Geometry check sheet. Reference: drawing and pictorial views, mm from the part's lowest x, y, z. A direction names the side the tool comes from. Round coordinates to 2 decimals unless told otherwise and drop trailing zeros. Order: outer loops, then holes, each group sorted by start corner. A loop starts at its lowest first (then second) coordinate and runs counter-clockwise, first axis right, second up.
(1) Tool access check on the marked faces 1 and 2. Record the directions out of +Z, -Z, +X, -X, +Y, -Y that give a thin tool (end or side, any length) a straight path to the whole face; none if there is none.
(2) Mould release check, pull along X, two halves, no side actions. Record for the marked faces 3, 4 and 5: released by +X, released by -X, zero draft, split by the parting line, or undercut.
(3) Thickness scan on probe 1 along X at (y, z) = (27, 8.5); probe 2 along Z at (x, y) = (1.15, 46.5); probe 3 along Y at (x, z) = (13, 3.25). Record the ranges inside material, lowest first.
(4) Sectioned sample at C-C, the plane z = 17. Enter the section's corners in (x, y).
(5) Depth check by flat-ended pin: pin 1 (12 mm diameter, centred on x = 29, z = 3.5, fed in from -Y); pin 2 (3.5 mm diameter, centred on y = 57, z = 10.25, fed in from -X); pin 3 (6 mm diameter, centred on x = 13, z = 15, fed in from +Y). Enter the tip coordinate at first touch or a pass-through.
(6) Sectioned sample at D-D, the plane y = 15.5. Enter the section's corners in (x, z).
(7) Sectioned sample at B-B, the plane y = 23.5. Enter the section's corners in (x, z), and give its area (3 significant figures).
(8) Sectioned sample at A-A, the plane y = 57. Enter the section's corners in (x, z) (3 decimals).
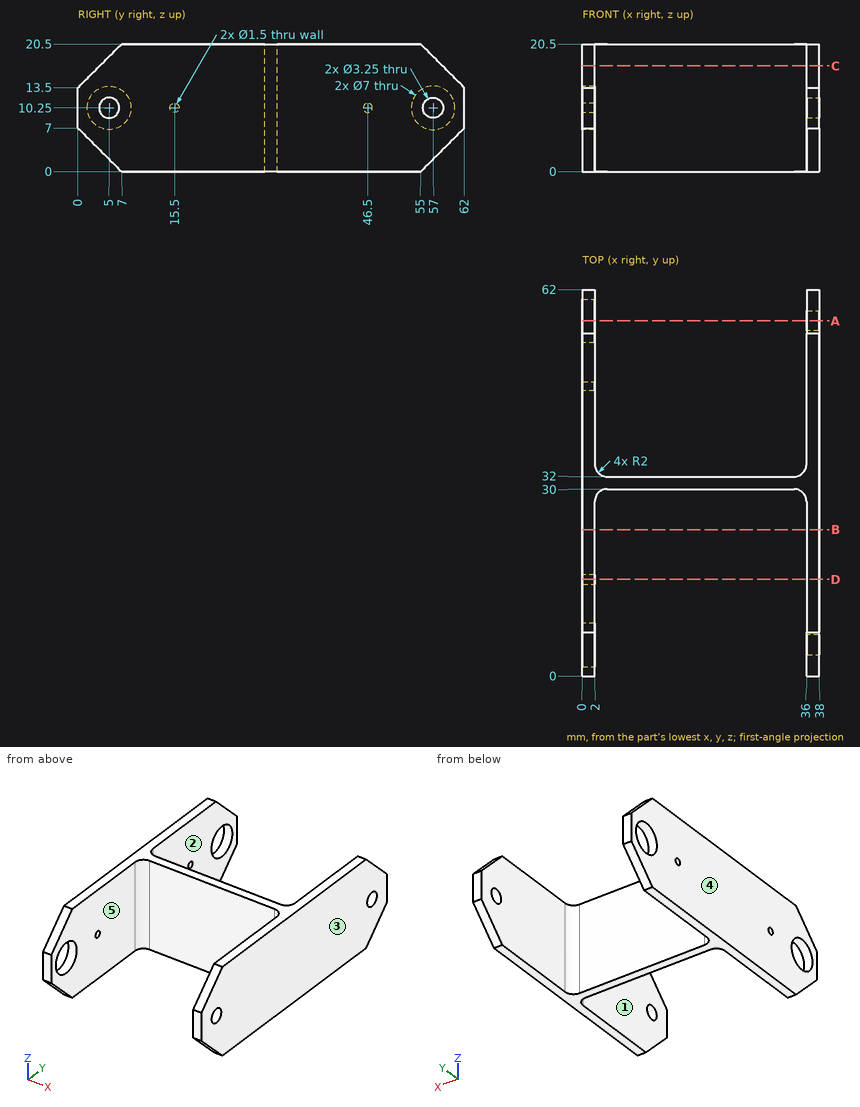
Derived:
1. face 1: +Z, -Z, -Y
1. face 2: +Z, -Z, +Y
2. face 3: released by +X
2. face 4: released by -X
2. face 5: undercut
3. probe 1: x = 0 to 2, 36 to 38
3. probe 2: z = 0 to 9.5, 11 to 20.5
3. probe 3: y = 30 to 32
4. outline: (0, 3.5) - (2, 3.5) - (2, 28) arc R2 cw to (4, 30) - (34, 30) arc R2 cw to (36, 28) - (36, 3.5) - (38, 3.5) - (38, 58.5) - (36, 58.5) - (36, 34) arc R2 cw to (34, 32) - (4, 32) arc R2 cw to (2, 34) - (2, 58.5) - (0, 58.5) - close
5. pin 1: stops at y = 29.73
5. pin 2: stops at x = 36
5. pin 3: stops at y = 32
6. outline: (0, 0) - (2, 0) - (2, 9.5) - (0, 9.5) - close; (0, 11) - (2, 11) - (2, 20.5) - (0, 20.5) - close; (36, 0) - (38, 0) - (38, 20.5) - (36, 20.5) - close
7. outline: (0, 0) - (2, 0) - (2, 20.5) - (0, 20.5) - close; (36, 0) - (38, 0) - (38, 20.5) - (36, 20.5) - close
7. area: 82.0 mm2
8. outline: (0, 2) - (2, 2) - (2, 6.75) - (0, 6.75) - close; (0, 13.75) - (2, 13.75) - (2, 18.5) - (0, 18.5) - close; (36, 2) - (38, 2) - (38, 8.625) - (36, 8.625) - close; (36, 11.875) - (38, 11.875) - (38, 18.5) - (36, 18.5) - close
